For this review, take the finished solid that the model builds, in its own axes (mm). A direction names the side the tool comes from. Coordinates: 2 decimals unless noted, no trailing zeros. Write each loop counter-clockwise with the first axis right and the second up, starting at its lowest first coordinate (ties: lowest second). Pieces come first, ordered by that corner, then holes. Notation, with made-up numbers: M 59,-1.5 L 82,-1.5 A4 ccw 82,4.5 Z; hole C 80,59.5 d1. An arc over 180 degrees is marked long. One line per question, with ' | ' between items.
from build123d import *

# Parameters (mm, degrees)
F0_W     = 94.106388
F0_H     = 83.2
F1_DEPTH = 6
F3_DEPTH = 6.001
F5_DEPTH = 6


with BuildPart() as f1:
    # F0 (on Top) → F1 (new body)
    with BuildSketch(Plane.XY):
        with Locations((47.053194, 41.6)):
            Rectangle(F0_W, F0_H)
        Polygon((67.404791, 6.35), (26.701597, 6.35), (6.35, 41.6), (26.701597, 76.85), (67.404791, 76.85), (87.756388, 41.6), align=None, mode=Mode.SUBTRACT)
    extrude(amount=F1_DEPTH)

    # F2 (on face) → F3 (cut, through all)
    with BuildSketch(Plane.XY.offset(6)):
        Polygon((0, 83.2), (0, 43.301477), (23.035423, 83.2), align=None)
        Polygon((94.106388, 83.2), (71.070965, 83.2), (94.106388, 43.301477), align=None)
        Polygon((94.106388, 39.898523), (71.070965, 0), (94.106388, 0), align=None)
        Polygon((23.035423, 0), (0, 39.898523), (0, 0), align=None)
    extrude(amount=-F3_DEPTH, mode=Mode.SUBTRACT)

    # F4 (on face) → F5 (join)
    with BuildSketch(Plane.XY.offset(6)):
        Polygon((23.035423, 0), (0, 39.898523), (29.44789, -32.987564), (29.553194, -103.15), (64.553194, -103.15), (64.658498, -32.987564), (94.106388, 39.898523), (71.070965, 0), align=None)
    extrude(amount=-F5_DEPTH)


solid = f1.part
1) To check wall thickness, follow line 1 along Y through (x, z) = (61, 1.7); line 2 along Y through (x, z) = (7.5, 1.6); line 3 along X through (y, z) = (-42.5, 3.1). State the ranges of each line that lie inside material, in increasing order. Write a range as [from, to].
Responses:
line 1: [-103.15, 6.35], [76.85, 83.2] | line 2: [21.34, 39.61], [43.59, 56.29] | line 3: [29.46, 64.64]
2) Machinability: for faces 4 (the flat face through (11.356, 62.971, 3.042)), 5 (the flat face through (16.668, 23.728, 2.958)), which of the approach directions +Z, -Z, +X, -X, +Y, -Y give a long, thin tool a straight path to every point of the face, cutting with its end or side? Answer none if there is none.
Responses:
face 4: +Z, -Z, -X, +Y | face 5: +Z, -Z
3) We need section B-B on z = 3.4. State the section outline as (x, y) points, then the cut area to 3 significant figures.
Responses:
outline: M 0,39.9 L 29.45,-32.99 L 29.55,-103.15 L 64.55,-103.15 L 64.66,-32.99 L 94.11,39.9 L 94.11,43.3 L 71.07,83.2 L 23.04,83.2 L 0,43.3 Z; hole M 6.35,41.6 L 26.7,6.35 L 67.4,6.35 L 87.76,41.6 L 67.4,76.85 L 26.7,76.85 Z | area: 6,030 mm^2
4) We need section D-D on y = -41.5. State the section outline as (x, z) points, then the cut area to 3 significant figures.
Responses:
outline: M 29.46,0 L 64.65,0 L 64.65,6 L 29.46,6 Z | area: 211 mm^2
5) We need section C-C on y = 65.5. State the section outline as (x, z) points.
Responses:
outline: M 12.82,0 L 20.15,0 L 20.15,6 L 12.82,6 Z; M 73.96,0 L 81.29,0 L 81.29,6 L 73.96,6 Z
6) The part is to be moulded in two halves that separate along X. For faces 1 (the flat face through (47, 83.2, 3)), 2 (the flat face through (14.518, 3.966, 3.042)), 3 (the flat face through (47, 6.35, 3)), say which applies: +X half, -X half, draft (parallel to the pull), parting line (faces both ways), or undercut.
Responses:
face 1: draft | face 2: -X half | face 3: undercut
7) Insertion check: pin 1 Ø1 at (x, z) = (21, 5) entering from +Y; pin 2 Ø1.5 at (y, z) = (-40, 4.5) entering from -X; pin 3 Ø2 at (y, z) = (18, 5.5) entering from +X. Each pin has a flat end and moves straight along its axis. Give the tip position at first contact, or say it passes through.
Responses:
pin 1: y = 80.54 | pin 2: x = 29.46 | pin 3: x = 85.66
8) We need section A-A on x = 45. State the section outline as (y, z) points.
Responses:
outline: M -103.15,0 L 6.35,0 L 6.35,6 L -103.15,6 Z; M 76.85,0 L 83.2,0 L 83.2,6 L 76.85,6 Z
